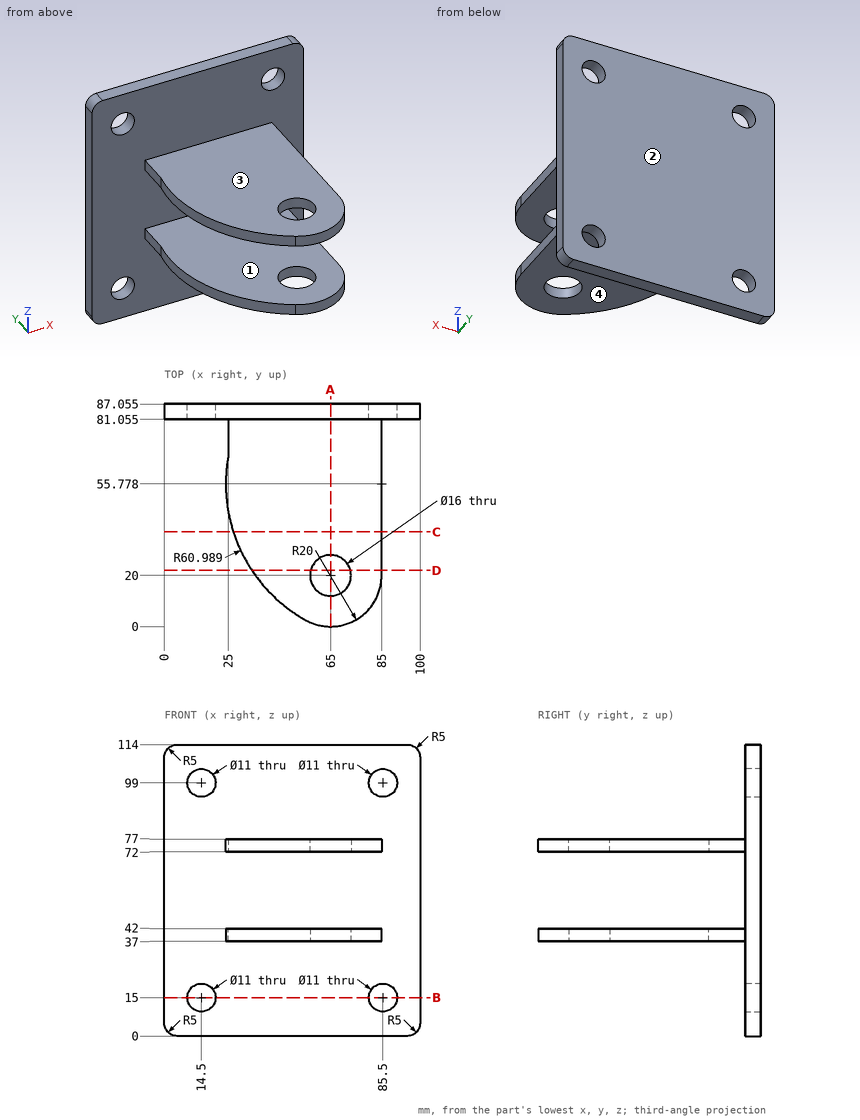
The figure shows three views and two pictorial views of one solid part (mm, origin at its lowest corner). Answer the questions. Round coordinates to 2 decimals unless told otherwise and drop trailing zeros. Write each loop counter-clockwise with the first axis right and the second up, starting at its lowest first coordinate (ties: lowest second). Pieces come first, ordered by that corner, then holes. Notation, with made-up numbers: (28.25, 54) - (65.25, 54) arc R21 ccw to (65.25, 71) - close; hole circle Ø9 at (-9, -36.5). An arc over 180 degrees is marked (long way). Use one line per item in the form item = value. Start each with the question number.
Item 1: Determine the mould class of the marked faces 1, 2, 3 and 4 for opening direction Z: +Z half, -Z half, draft (parallel to the pull), parting line (faces both ways), or undercut.
Item 2: Flat-ended cylindrical pins translate along their axes: pin 1 Ø2.5 at (y, z) = (47, 75) entering from +X; pin 2 Ø4 at (y, z) = (71, 38.5) entering from -X; pin 3 Ø6 at (x, y) = (76.5, 59.5) entering from -Z. Find the tip coordinate at first contact, or state that the pin passes through.
Item 3: A cutting plane is placed at B-B (z = 15). Write down the section's boundary in (x, y) (1 decimal).
Item 4: Find the intervals of material crossed by line 1 (X direction, y = 83, z = 99); line 2 (Z direction, x = 14, y = 85); line 3 (Z direction, x = 75.5, y = 45.5), in increasing order. Write a range as [from, to].
Item 5: A cutting plane is placed at C-C (y = 37). Write down the section's boundary in (x, z), plus the area to 3 significant figures.
Item 6: A cutting plane is placed at A-A (x = 65). Write down the section's boundary in (y, z) (1 decimal).
Item 7: A cutting plane is placed at D-D (y = 22). Write down the section's boundary in (x, z).
The answers:
q1.face_1 = undercut
q1.face_2 = draft
q1.face_3 = +Z half
q1.face_4 = -Z half
q2.pin_1 = 85
q2.pin_2 = 25
q2.pin_3 = 37
q3.outline = (0, 81.1) - (9, 81.1) - (9, 87.1) - (0, 87.1) - close; (20, 81.1) - (80, 81.1) - (80, 87.1) - (20, 87.1) - close; (91, 81.1) - (100, 81.1) - (100, 87.1) - (91, 87.1) - close
q4.line_1 = [0, 9], [20, 80], [91, 100]
q4.line_2 = [0, 9.52], [20.48, 93.52], [104.48, 114]
q4.line_3 = [37, 42], [72, 77]
q5.outline = (26.97, 37) - (85, 37) - (85, 42) - (26.97, 42) - close; (26.97, 72) - (85, 72) - (85, 77) - (26.97, 77) - close
q5.area = 580 mm^2
q6.outline = (0, 37) - (12, 37) - (12, 42) - (0, 42) - close; (0, 72) - (12, 72) - (12, 77) - (0, 77) - close; (28, 37) - (81.1, 37) - (81.1, 0) - (87.1, 0) - (87.1, 114) - (81.1, 114) - (81.1, 77) - (28, 77) - (28, 72) - (81.1, 72) - (81.1, 42) - (28, 42) - close
q7.outline = (34.22, 37) - (57.25, 37) - (57.25, 42) - (34.22, 42) - close; (34.22, 72) - (57.25, 72) - (57.25, 77) - (34.22, 77) - close; (72.75, 37) - (85, 37) - (85, 42) - (72.75, 42) - close; (72.75, 72) - (85, 72) - (85, 77) - (72.75, 77) - close
